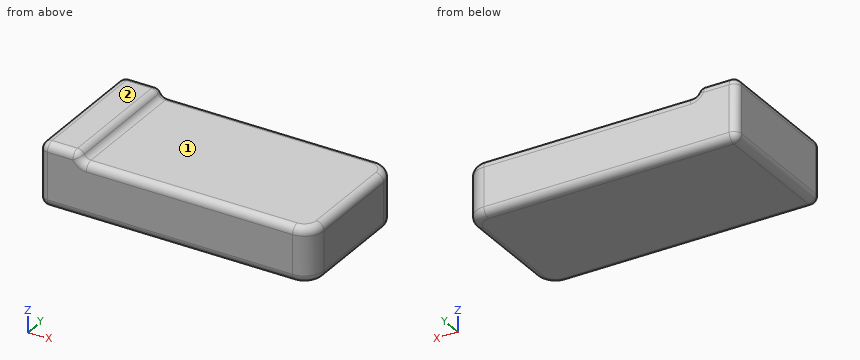
```python
from build123d import *

# Parameters (mm, degrees)
F1_DEPTH = 35
F2_R     = 5
F3_R     = 2


with BuildPart() as f1:
    # F0 (on Front) → F1 (new body)
    with BuildSketch(Plane.XZ):
        with BuildLine():
            Line((-19.8307685554, 3.7411112362), (-29.8307685554, 3.7411112362))
            Line((-29.8307685554, 3.7411112362), (-29.8307685554, -12.2588887638))
            Line((-29.8307685554, -12.2588887638), (40.1692314446, -12.2588887638))
            Line((40.1692314446, -12.2588887638), (40.1692314446, 1.7411112362))
            Line((40.1692314446, 1.7411112362), (-17.8307685554, 1.7411112362))
            ThreePointArc((-17.8307685554, 1.7411112362), (-19.2449821178, 2.3268976739), (-19.8307685554, 3.7411112362))
        make_face()
    extrude(amount=F1_DEPTH)

    # F2
    f2_edges = [f1.edges().sort_by_distance(p)[0] for p in [
        (40.169231, -35, -5.258889),
        (40.169231, 0, -5.258889),
    ]]
    fillet(f2_edges, radius=F2_R)

    # F3
    f3_edges = [f1.edges().sort_by_distance(p)[0] for p in [
        (-19.830769, -17.5, 3.741111),
        (-29.830769, -17.5, 3.741111),
        (-24.830769, 0, 3.741111),
        (-24.830769, -35, 3.741111),
        (2.669231, -35, -12.258889),
        (35.169231, -35, -5.258889),
        (-29.830769, -35, -4.258889),
        (8.669231, -35, 1.741111),
        (-19.244982, -35, 2.326898),
        (2.669231, 0, -12.258889),
        (35.169231, 0, -5.258889),
        (-29.830769, 0, -4.258889),
        (8.669231, 0, 1.741111),
        (-19.244982, 0, 2.326898),
        (-29.830769, -17.5, -12.258889),
    ]]
    fillet(f3_edges, radius=F3_R)


solid = f1.part
```
Geometry check sheet. Reference: the model listing, model coordinates, mm. Face numbers are marked on the shaded views. A direction names the side the tool comes from. Give positions to 0.01 mm unless a question says otherwise; leave off trailing zeros. Order: outer loops, then holes, each group sorted by start corner. A loop starts at its lowest first (then second) coordinate and runs counter-clockwise, first axis right, second up. Notation, with made-up numbers: (-24.5, 20.5) - (-15.5, 20.5) arc R31 cw to (-15.5, 59.5) - close; hole circle Ø8 at (87, 24). An arc over 180 degrees is marked (long way). Answer in a Markdown table with one row per item. Add a question column.
Q1. Tool access check on the marked faces 1 and 2. Record the directions out of +Z, -Z, +X, -X, +Y, -Y that give a thin tool (end or side, any length) a straight path to the whole face; none if there is none.
Q2. Material ranges on probe 1 along Z at (x, y) = (35, -27.5); probe 2 along X at (y, z) = (-18.5, 1.25); probe 3 along Y at (x, z) = (-13, 0), recorded low to high. Write a range as from..to.
Q3. Gauge pin test, flat end, axial feed: pin 1 (10 mm diameter, centred on x = 1.5, y = -18, fed in from +Z). Record the tip position at first contact, or that the pin passes through.
Q4. Cross-section at B-B, the plane y = -6. Enter the section's corners in (x, z), then the cut area to 3 significant figures.
Q5. Cross-section at A-A, the plane x = 34.5. Enter the section's corners in (y, z), then the cut area to 3 significant figures.
Check values:
| question | item | result |
|---|---|---|
| 1 | face 1 | +Z, +X, +Y, -Y |
| 1 | face 2 | +Z, +X, -X, +Y, -Y |
| 2 | probe 1 | z = -12.26..1.74 |
| 2 | probe 2 | x = -29.83..39.48 |
| 2 | probe 3 | y = -34.98..-0.02 |
| 3 | pin 1 | stops at z = 1.74 |
| 4 | outline | (-29.83, -10.26) arc R2 ccw to (-27.83, -12.26) - (38.17, -12.26) arc R2 ccw to (40.17, -10.26) - (40.17, -0.26) arc R2 ccw to (38.17, 1.74) - (-17.83, 1.74) arc R2 cw to (-19.56, 2.74) arc R2 ccw to (-21.29, 3.74) - (-27.83, 3.74) arc R2 ccw to (-29.83, 1.74) - close |
| 4 | area | 997 mm^2 |
| 5 | outline | (-35, -10.26) arc R2 ccw to (-33, -12.26) - (-2, -12.26) arc R2 ccw to (0, -10.26) - (0, -0.26) arc R2 ccw to (-2, 1.74) - (-33, 1.74) arc R2 ccw to (-35, -0.26) - close |
| 5 | area | 487 mm^2 |
